from build123d import *

# Parameters (mm, degrees)
ESBO_O1_W                = 130
ESBO_O1_H                = 50
RESSALTO_EXTRUS_O1_DEPTH = 15
ESBO_O2_W                = 110
ESBO_O2_H                = 10
CORTE_EXTRUS_O1_DEPTH    = 51
ESBO_O5_R                = 2
CORTE_EXTRUS_O2_DEPTH    = 10
CORTE_EXTRUS_O3_START    = -10
ESBO_O6_R                = 2
CORTE_EXTRUS_O3_DEPTH    = 10
ESBO_O7_R                = 2
CORTE_EXTRUS_O4_DEPTH    = 10
CORTE_EXTRUS_O5_START    = -10
ESBO_O8_R                = 2
CORTE_EXTRUS_O5_DEPTH    = 10
ESBO_O13_R               = 1.5
ESBO_O13_R_2             = 5
CORTE_EXTRUS_O8_DEPTH    = 10
ESBO_O14_R               = 1.5
ESBO_O14_W               = 18.4
ESBO_O14_H               = 11.1
CORTE_EXTRUS_O9_DEPTH    = 10


with BuildPart() as part:
    # Esboço1 → Ressalto-extrusão1 (new body)
    with BuildSketch(Plane(origin=(0, 0, 0), x_dir=(1, 0, 0), z_dir=(0, 1, 0))):
        with Locations((-65, 25)):
            Rectangle(ESBO_O1_W, ESBO_O1_H)
    extrude(amount=RESSALTO_EXTRUS_O1_DEPTH)

    # Esboço2 → Corte-extrusão1 (cut)
    with BuildSketch(Plane(origin=(0, 0, -50), x_dir=(-1, 0, 0), z_dir=(0, 0, -1))):
        with Locations((65, 5)):
            Rectangle(ESBO_O2_W, ESBO_O2_H)
    extrude(amount=-CORTE_EXTRUS_O1_DEPTH, mode=Mode.SUBTRACT)

    # Esboço5 → Corte-extrusão2 (cut)
    with BuildSketch(Plane(origin=(0, 0, -50), x_dir=(-1, 0, 0), z_dir=(0, 0, -1))):
        with Locations((125, 5)):
            Circle(ESBO_O5_R)
        with Locations((5, 5)):
            Circle(ESBO_O5_R)
    extrude(amount=-CORTE_EXTRUS_O2_DEPTH, mode=Mode.SUBTRACT)

    # Esboço6 → Corte-extrusão3 (cut)
    with BuildSketch(Plane.XY.offset(CORTE_EXTRUS_O3_START)):
        with Locations(Location((-125, 5, 0), (0, 0, 180))):
            Circle(ESBO_O6_R)
        with Locations(Location((-5, 5, 0), (0, 0, 180))):
            Circle(ESBO_O6_R)
    extrude(amount=CORTE_EXTRUS_O3_DEPTH, mode=Mode.SUBTRACT)

    # Esboço7 → Corte-extrusão4 (cut)
    with BuildSketch(Plane(origin=(0, 0, 0), x_dir=(0, 0, -1), z_dir=(1, 0, 0))):
        with Locations((25, 5)):
            Circle(ESBO_O7_R)
    extrude(amount=-CORTE_EXTRUS_O4_DEPTH, mode=Mode.SUBTRACT)

    # Esboço8 → Corte-extrusão5 (cut)
    with BuildSketch(Plane.ZY.offset(130).offset(CORTE_EXTRUS_O5_START)):
        with Locations(Location((-25, 5, 0), (0, 0, 180))):
            Circle(ESBO_O8_R)
    extrude(amount=CORTE_EXTRUS_O5_DEPTH, mode=Mode.SUBTRACT)

    # Esboço13 → Corte-extrusão8 (cut)
    with BuildSketch(Plane(origin=(0, 15, 0), x_dir=(1, 0, 0), z_dir=(0, 1, 0))):
        with Locations(Location((-115, 35, 0), (0, 0, 270))):
            Circle(ESBO_O13_R)
        with Locations(Location((-100, 35, 0), (0, 0, 270))):
            Circle(ESBO_O13_R_2)
        with Locations(Location((-85, 35, 0), (0, 0, 270))):
            Circle(ESBO_O13_R)
    extrude(amount=-CORTE_EXTRUS_O8_DEPTH, mode=Mode.SUBTRACT)

    # Esboço14 → Corte-extrusão9 (cut)
    with BuildSketch(Plane(origin=(0, 15, 0), x_dir=(1, 0, 0), z_dir=(0, 1, 0))):
        with Locations(Location((-68, 33.75, 0), (0, 0, 270))):
            Circle(ESBO_O14_R)
        with Locations(Location((-43, 33.75, 0), (0, 0, 270))):
            Circle(ESBO_O14_R)
        with Locations((-55.5, 33.75)):
            Rectangle(ESBO_O14_W, ESBO_O14_H)
    extrude(amount=-CORTE_EXTRUS_O9_DEPTH, mode=Mode.SUBTRACT)


solid = part.part
Work out the finished part from the listing and answer in its coordinate system (mm). A direction names the side the tool comes from. Coordinates: 2 decimals unless noted, no trailing zeros. Write each loop counter-clockwise with the first axis right and the second up, starting at its lowest first coordinate (ties: lowest second). Pieces come first, ordered by that corner, then holes. Notation, with made-up numbers: M -5.75,59.25 L 39.25,59.25 A13 ccw 39.25,72.25 Z; hole C -7,45.25 d4. An arc over 180 degrees is marked long. Write item = value, one per line.
1. Flat-ended cylindrical pins translate along their axes: pin 1 (4 mm diameter, centred on x = -85, z = -35, fed in from -Y); pin 2 (2.5 mm diameter, centred on x = -125, y = 5, fed in from -Z); pin 3 (6 mm diameter, centred on x = -93, y = 10, fed in from +Z). Find the tip coordinate at first contact, or state that the pin passes through.
Solution:
pin_1 = 10
pin_2 = -40
pin_3 = 0
2. The part is cut by section B-B (x = -5). Determine the outline of the cut face in (y, z).
Solution:
outline = M 0,-50 L 3,-50 L 3,-40 L 7,-40 L 7,-50 L 15,-50 L 15,0 L 7,0 L 7,-10 L 3,-10 L 3,0 L 0,0 Z; hole C 5,-25 d4
3. The part is cut by section D-D (x = -85). Determine the outline of the cut face in (y, z).
Solution:
outline = M 10,-50 L 15,-50 L 15,-36.5 L 10,-36.5 Z; M 10,-33.5 L 15,-33.5 L 15,0 L 10,0 Z
4. Straight lines are drawn through the part: line 1 (X direction, y = 5, z = -2.75); line 2 (Y direction, x = -126, z = -25); line 3 (X direction, y = 9.75, z = -47). For each, find the intervals that lie inside material, in ascending order. Write a range as from..to.
Solution:
line_1 = -130..-127, -123..-120, -10..-7, -3..0
line_2 = 0..3, 7..15
line_3 = -130..-120, -10..0
5. Determine the mould class of faces 5 (the face through (-123, 5, -5)), 6 (the face through (0, 7.4, -24.7)), 7 (the face through (-125, 0, -25)) for opening direction Y: released by +Y, released by -Y, zero draft, split by the parting line, or undercut.
Solution:
face_5 = undercut
face_6 = zero draft
face_7 = released by -Y
6. The part is cut by section A-A (z = -6). Determine the outline of the cut face in (x, y).
Solution:
outline = M -130,0 L -120,0 L -120,10 L -10,10 L -10,0 L 0,0 L 0,15 L -130,15 Z; hole C -125,5 d4; hole C -5,5 d4
7. For faces 1 (the face through (-10, 7.2, -25.4)), 2 (the face through (-125, 5, -10)), 3 (the face through (-66, 15, -25)), 4 (the face through (-46.3, 13, -34)), determine the directions among +Z, -Z, +X, -X, +Y, -Y from which every point of the face is accessible in a straight line to the end or side of a thin tool.
Solution:
face_1 = +Z, -Z, -Y
face_2 = +Z
face_3 = +Z, -Z, +X, -X, +Y
face_4 = +Y, -Y
8. The part is cut by section C-C (y = 1.5). Determine the outline of the cut face in (x, z), then the cut area to 3 significant figures.
Solution:
outline = M -130,-50 L -120,-50 L -120,0 L -130,0 Z; M -10,-50 L 0,-50 L 0,0 L -10,0 Z
area = 1,000 mm2
